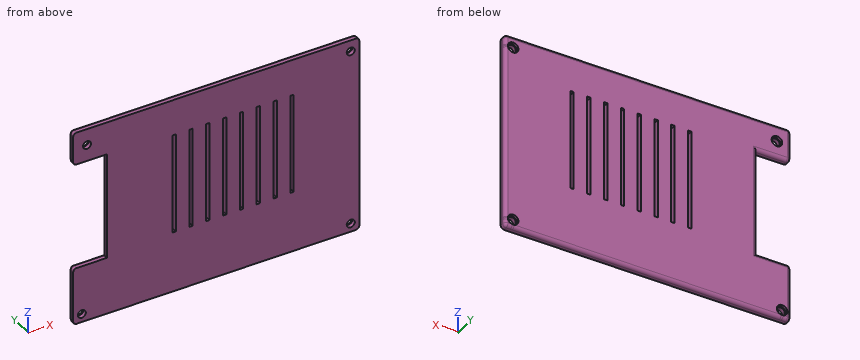
Autodesk Inventor part; units mm, degrees
ref_plane "YZ Plane" through (0, 0, 0) normal (1, 0, 0) x (0, 1, 0)
ref_plane "XZ Plane" through (0, 0, 0) normal (0, 1, 0) x (-1, 0, 0)
ref_plane "XY Plane" through (0, 0, 0) normal (0, 0, 1) x (1, 0, 0)
sketch "Sketch1" plane through (0, 0, 0) normal (0, 1, 0) x (-1, 0, 0)
  line L0 (22, -33) -> (-148, -33)
  line L1 (22, 2) -> (22, -33)
  line L2 (2, 2) -> (22, 2)
  line L3 (2, 67) -> (2, 2)
  line L4 (22, 67) -> (2, 67)
  line L5 (22, 87) -> (22, 67)
  line L6 (-148, 87) -> (22, 87)
  line L7 (-148, -33) -> (-148, 87)
  circle A0 centre (16.9, -27.9) radius 2.4
  circle A1 centre (13.8, 77) radius 2.4
  arc A2 (-145.3101, 79.6937) -> (-145.3101, 80.5063) centre (-142.9447, 80.1) ccw
  arc A3 (-142.9447, -30.3) -> (-145.3101, -27.4937) centre (-142.9447, -27.9) ccw
  circle A4 centre (-142.9447, -27.9) radius 2.4
  circle A5 centre (-142.9447, 80.1) radius 2.4
  point P0 (0, 0)
  point P1 (22, -33)
extrude "Extrusion1" add sketch "Sketch1" along normal blind 4
extrude "Extrusion2" add sketch "Sketch1" along normal blind 30 contours A0 | A1 | A5 A2 | A4 A3
fillet "Fillet1" radius 1 4 edges at (-11.4, 30, 77) (-14.5, 30, -27.9) (140.5794, 30, -28.3063) (140.5794, 30, 79.6937)
sketch "Sketch2" plane through (0, 4, 0) normal (0, 1, 0) x (1, 0, 0)
  circle A0 centre (-16.9, 27.9) radius 2.4
  circle A1 centre (142.9447, 27.9) radius 2.4
  circle A2 centre (142.9447, -80.1) radius 2.4
  circle A3 centre (-13.8, -77) radius 2.4
  point P0 (0, 0)
extrude "Extrusion3" cut sketch "Sketch2" along normal through all both and the other way through all
sketch "Sketch3" plane through (0, 0, 0) normal (0, -1, 0) x (1, 0, 0)
  line L0 (37, 65) -> (39, 65)
  line L1 (39, 65) -> (39, 4)
  line L2 (39, 4) -> (37, 4)
  line L3 (37, 4) -> (37, 65)
  point P0 (0, 0)
extrude "Extrusion4" cut sketch "Sketch3" against normal through all
pattern_linear "Rectangular Pattern1" count 8 spacing 10 along (1, 0, 0) of "Extrusion4"
sketch "Sketch4" plane through (0, 4, 0) normal (0, 1, 0) x (1, 0, 0)
  circle A0 centre (-16.9, 27.9) radius 2.4
  circle A1 centre (142.9447, 27.9) radius 2.4
  circle A2 centre (142.9447, -80.1) radius 2.4
  circle A3 centre (-13.8, -77) radius 2.4
  circle A4 centre (-16.9, 27.9) radius 3.15
  circle A5 centre (142.9447, 27.9) radius 3.15
  circle A6 centre (142.9447, -80.1) radius 3.15
  circle A7 centre (-13.8, -77) radius 3.15
  point P0 (0, 0)
  dimension "d16" = 0.75
  dimension "d17" = 0.75
  dimension "d18" = 0.75
  dimension "d19" = 0.75
extrude "Extrusion5" cut sketch "Sketch4" against normal blind 1.5 contours A0 | A1 | A2 | A3 | A4 | A5 | A6 | A7
fillet "Fillet2" radius 2 6 edges at (-22, 2, 67) (-22, 2, -33) (-22, 2, 2) (148, 2, -33) (148, 2, 87) (-22, 2, 87)
fillet "Fillet3" radius 2 14 edges at (-2, 4, 34.5) (-21.4142, 4, 1.4142) (-11, 4, 2) (-21.4142, 4, -32.4142) (63, 4, -33) (147.4142, 4, -32.4142) (148, 4, 27) (147.4142, 4, 86.4142) (63, 4, 87) (-21.4142, 4, 86.4142) (-22, 4, 77) (-21.4142, 4, 67.5858) (-11, 4, 67) (-22, 4, -15.5)
properties material "ABS Plastic"
Part model, mm, in its own coordinate system. Round coordinates to 2 decimals unless told otherwise and drop trailing zeros.
1. Slice it at A-A (z = 45). Count the separate pieces of the cut face and the enclosed holes in it, and give its area (3 significant figures).
Solutions:
separate pieces: 9
enclosed holes: 0
area: 534 mm2
2. Flat gauge pins, fed straight in: pin 1 (2 mm diameter, centred on y = 3, z = 41.5, fed in from +X); pin 2 (1.2 mm diameter, centred on y = 2.5, z = 34, fed in from -X); pin 3 (5 mm diameter, centred on x = -17, z = -28, fed in from +Y); pin 4 (0.6 mm diameter, centred on x = 97.5, y = 3, fed in from -Z). Where does each tip first touch, or does it go through?
Solutions:
pin 1: stops at x = 148
pin 2: stops at x = -2
pin 3: stops at y = 2.5
pin 4: stops at z = -32.87
3. Drill centre lines: line 1 along X through (y, z) = (0.8, -27.9); line 2 along X through (y, z) = (3.8, 79); line 3 along X through (y, z) = (0.9, 77). Where is each one in solid material? Low to high.
Solutions:
line 1: x = -22 to -19.3, -14.5 to 140.54, 145.34 to 148
line 2: x = -20.87 to -16.23, -11.37 to 139.99, 145.9 to 146.87
line 3: x = -22 to -16.2, -11.4 to 148
